```python
from build123d import *

# Parameters (mm, degrees)
CUT_EXTRUDE1_DEPTH = 4


with BuildPart() as part:
    # Sketch1 → Revolve1 (revolve)
    with BuildSketch(Plane(origin=(0, 0, 0), x_dir=(0, 0, -1), z_dir=(1, 0, 0)), mode=Mode.PRIVATE) as revolve1_sk:
        Polygon((-4, 0), (-4, 4), (110.3, 4), (110.3, 10), (115.3, 10), (115.3, 0), align=None)
    revolve(revolve1_sk.sketch.rotate(Axis((0, 0, -115.3), (0, 0, 1)), 270), axis=Axis((0, 0, -115.3), (0, 0, 1)))

    # Sketch2 → Revolve2 (revolve)
    with BuildSketch(Plane(origin=(0, 0, 0), x_dir=(0, 0, -1), z_dir=(1, 0, 0)), mode=Mode.PRIVATE) as revolve2_sk:
        with BuildLine():
            Line((-24, 0), (-24, 3.233))
            Line((-24, 3.233), (-23.233, 4))
            Line((-23.233, 4), (-7.697981936, 4))
            Line((-7.697981936, 4), (-5.599415898, 3.236184428))
            ThreePointArc((-5.599415898, 3.236184428), (-5.498392718, 3.209115348), (-5.394203812, 3.2))
            Line((-5.394203812, 3.2), (-4.6, 3.2))
            ThreePointArc((-4.6, 3.2), (-4.175735931, 3.375735931), (-4, 3.8))
            Line((-4, 3.8), (-4, 4))
            Line((-4, 4), (-3, 4))
            Line((-3, 4), (-3, 0))
            Line((-3, 0), (-24, 0))
        make_face()
    revolve(revolve2_sk.sketch.rotate(Axis((0, 0, 3), (0, 0, 1)), 270), axis=Axis((0, 0, 3), (0, 0, 1)))

    # Sketch3 → Cut-Extrude1 (cut)
    with BuildSketch(Plane.XY.offset(1)):
        Polygon((-7, 14), (-7, -7), (-3.5, -7), (-3.5, 7), (3.5, 7), (3.5, -7), (7, -7), (7, 14), align=None)
    extrude(amount=CUT_EXTRUDE1_DEPTH, mode=Mode.SUBTRACT)


solid = part.part
```
Could you check a few things on this model? Use its own coordinates, in mm. A direction names the side the tool comes from. Round coordinates to 2 decimals unless told otherwise and drop trailing zeros. Loops run counter-clockwise (first coordinate to the right, second up) from the corner with the lowest first, then second, coordinate; pieces in that order, holes last. Notation, with made-up numbers: (62.5, 83) - (101.5, 83) arc R9 ccw to (101.5, 94) - close; hole circle Ø9 at (38.25, -39). An arc over 180 degrees is marked (long way). Use CSV: the item, a comma, the result in double quotes.
Item 1: If we section it at A-A on x = 0: List the corners of the cut face in (y, z) for me, then the cut area to 3 significant figures.
Here are the results:
outline,"(-10, -115.3) - (10, -115.3) - (10, -110.3) - (4, -110.3) - (4, 4) - (3.8, 4) arc R0.6 cw to (3.2, 4.6) - (3.2, 5.39) arc R0.6 cw to (3.24, 5.6) - (4, 7.7) - (4, 23.23) - (3.23, 24) - (-3.23, 24) - (-4, 23.23) - (-4, 7.7) - (-3.24, 5.6) arc R0.6 cw to (-3.2, 5.39) - (-3.2, 4.6) arc R0.6 cw to (-3.8, 4) - (-4, 4) - (-4, -110.3) - (-10, -110.3) - close"
area,"1,170 mm²"
Item 2: Will these pins go through, and if not, where does the flat tip stop? pin 1 (8 mm diameter, centred on y = -7, z = -7.5, fed in from -X); pin 2 (3.5 mm diameter, centred on y = 0, z = 2.5, fed in from +X); pin 3 (10 mm diameter, centred on y = -1.5, z = -22, fed in from -X).
Here are the results:
pin 1,"stops at x = -2.65"
pin 2,"stops at x = 4"
pin 3,"stops at x = -4"
Item 3: For faces 4 (the flat face through (-4.3, 0.1, -110.3)), 5 (the flat face through (0, 0, 24)), 6 (the flat face through (3.5, 0, 3)), 7 (the cylindrical face through (-2.539, -1.947, 4.992)), 8 (the cylindrical face through (-2.17, -9.76, -112.84)), which set-ups out of +Z, -Z, +X, -X, +Y, -Y let a thin tool reach every point of the face, with its end or its side?
Here are the results:
face 4,"+Z"
face 5,"+Z, +X, -X, +Y, -Y"
face 6,"+X, +Y, -Y"
face 7,"none"
face 8,"+Z, -Z"
Item 4: If we mould it in two halves opening along Z, with no side actions, what happens to faces 1 (the cylindrical face through (-0.867, -3.905, -53.95)), 2 (the flat face through (-3.5, 0, 3)), 3 (the flat face through (0, 0, -115.3))? For each: pulls with the +Z half, pulls with the -Z half, needs draft (parallel to the pull), parting line crosses it, or undercut.
Here are the results:
face 1,"needs draft"
face 2,"undercut"
face 3,"pulls with the -Z half"
Item 5: I need wall thicknesses on L1, parallel to Z at x = -1.75, y = 4.75; L2, parallel to Y at x = 0.25, z = -35; L3, parallel to Y at x = 3, z = -68.5. Which ranges of each line are inside material? Lowest first, please. Write a range as [from, to].
Here are the results:
L1,"z = [-115.3, -110.3]"
L2,"y = [-3.99, 3.99]"
L3,"y = [-2.65, 2.65]"
Item 6: If we section it at B-B on y = 0: List the corners of the cut face in (x, z) for me, then the cut area to 3 significant figures.
Here are the results:
outline,"(-10, -115.3) - (10, -115.3) - (10, -110.3) - (4, -110.3) - (4, 1) - (3.5, 1) - (3.5, 4.08) arc R0.6 cw to (3.2, 4.6) - (3.2, 5.39) arc R0.6 cw to (3.24, 5.6) - (4, 7.7) - (4, 23.23) - (3.23, 24) - (-3.23, 24) - (-4, 23.23) - (-4, 7.7) - (-3.24, 5.6) arc R0.6 cw to (-3.2, 5.39) - (-3.2, 4.6) arc R0.6 cw to (-3.5, 4.08) - (-3.5, 1) - (-4, 1) - (-4, -110.3) - (-10, -110.3) - close"
area,"1,170 mm²"
Item 7: If we section it at C-C on z = -43.5: List the corners of the cut face in (x, y) for me.
Here are the results:
outline,"circle Ø8 at (0, 0)"
Item 8: If we section it at D-D on y = 8: List the corners of the cut face in (x, z) for me.
Here are the results:
outline,"(-6, -115.3) - (6, -115.3) - (6, -110.3) - (-6, -110.3) - close"
